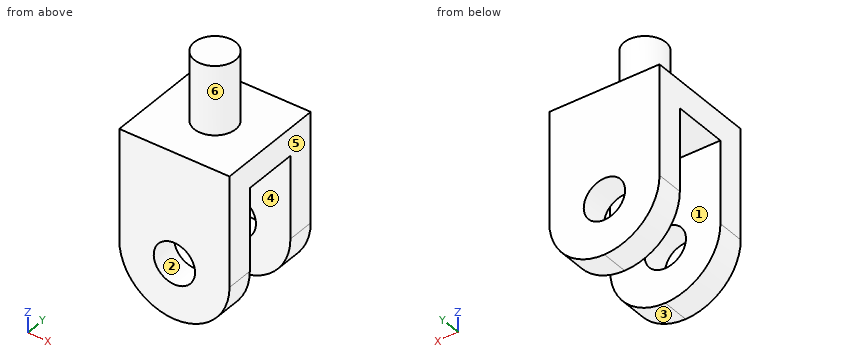
```python
from build123d import *

# Parameters (mm, degrees)
SKETCH1_W           = 16
SKETCH1_H           = 16
BOSS_EXTRUDE1_DEPTH = 24
SKETCH3_R           = 3
BOSS_EXTRUDE2_DEPTH = 10
SKETCH4_W           = 20
SKETCH4_H           = 8
CUT_EXTRUDE1_DEPTH  = 39.418745425
SKETCH5_R           = 3
CUT_EXTRUDE2_DEPTH  = 39.418745425
FILLET1_R           = 8


with BuildPart() as part:
    # Sketch1 → Boss-Extrude1 (new body)
    with BuildSketch(Plane.XY):
        Rectangle(SKETCH1_W, SKETCH1_H)
    extrude(amount=BOSS_EXTRUDE1_DEPTH)

    # Sketch3 → Boss-Extrude2 (add)
    with BuildSketch(Plane.XY.offset(24)):
        Circle(SKETCH3_R)
    extrude(amount=BOSS_EXTRUDE2_DEPTH)

    # Sketch4 → Cut-Extrude1 (cut, through all)
    with BuildSketch(Plane.ZY.offset(8)):
        with Locations((10, 0)):
            Rectangle(SKETCH4_W, SKETCH4_H)
    extrude(amount=-CUT_EXTRUDE1_DEPTH, mode=Mode.SUBTRACT)

    # Sketch5 → Cut-Extrude2 (cut, through all)
    with BuildSketch(Plane.XZ.offset(8)):
        with Locations(Location((0, 8, 0), (0, 0, 270))):
            Circle(SKETCH5_R)
    extrude(amount=-CUT_EXTRUDE2_DEPTH, mode=Mode.SUBTRACT)

    # Fillet1
    fillet1_edges = [part.edges().sort_by_distance(p)[0] for p in [
        (-8, 6, 0),
        (8, 6, 0),
        (8, -6, 0),
        (-8, -6, 0),
    ]]
    fillet(fillet1_edges, radius=FILLET1_R - 0.0001)  # a hair under: the kernel refuses the full size


solid = part.part
```
The model under review builds one solid part; all positions refer to its coordinate system, in mm. Face numbers are marked on the shaded views. A direction names the side the tool comes from. Round coordinates to 2 decimals unless told otherwise and drop trailing zeros. Write each loop counter-clockwise with the first axis right and the second up, starting at its lowest first coordinate (ties: lowest second). Pieces come first, ordered by that corner, then holes.
(1) Wall thickness on L1, parallel to X at y = 5.85, z = 8; L2, parallel to Y at x = 6, z = 6; L3, parallel to Z at x = -5, y = -2.75: over which ranges is each line inside the solid? List them lowest first.
(2) Machinability: for the marked faces 4, 5 and 6, which of the approach directions +Z, -Z, +X, -X, +Y, -Y give a long, thin tool a straight path to every point of the face, cutting with its end or side? Answer none if there is none.
(3) We need section C-C on z = 7.5. Give the boundary of the cut face in (x, y), and give its area (3 significant figures).
(4) Mouldability with a two-part tool opening along Z and no side actions: class the marked faces 1, 2 and 3 as +Z half, -Z half, draft (parallel to the pull), parting line (faces both ways), or undercut.
(5) Insertion check: pin 1 (7 mm diameter, centred on x = 0, z = 8, fed in from +Y); pin 2 (4 mm diameter, centred on x = -1.5, y = 1, fed in from -Z). Each pin has a flat end and moves straight along its axis. Give the tip position at first contact, or say it passes through.
(6) We need section D-D on x = -2.5. Give the boundary of the cut face in (y, z), and give its area (3 significant figures).
(7) We need section A-A on z = 2. Give the boundary of the cut face in (x, y), and give its area (3 significant figures).
Findings below:
1. L1: x = -8 to -3, 3 to 8
1. L2: y = -8 to -4, 4 to 8
1. L3: z = 20 to 24
2. face 4: -Z, +X, -X
2. face 5: +Z, -Z, +X, +Y, -Y
2. face 6: +Z
3. outline: (-7.98, -8) - (-2.96, -8) - (-2.96, -4) - (-7.98, -4) - close; (-7.98, 4) - (-2.96, 4) - (-2.96, 8) - (-7.98, 8) - close; (2.96, -8) - (7.98, -8) - (7.98, -4) - (2.96, -4) - close; (2.96, 4) - (7.98, 4) - (7.98, 8) - (2.96, 8) - close
3. area: 80.4 mm2
4. face 1: draft
4. face 2: undercut
4. face 3: -Z half
5. pin 1: stops at y = 8
5. pin 2: stops at z = 20
6. outline: (-8, 0.4) - (-4, 0.4) - (-4, 6.34) - (-8, 6.34) - close; (-8, 9.66) - (-4, 9.66) - (-4, 20) - (4, 20) - (4, 9.66) - (8, 9.66) - (8, 24) - (1.66, 24) - (1.66, 34) - (-1.66, 34) - (-1.66, 24) - (-8, 24) - close; (4, 0.4) - (8, 0.4) - (8, 6.34) - (4, 6.34) - close
6. area: 227 mm2
7. outline: (-5.29, -8) - (5.29, -8) - (5.29, -4) - (-5.29, -4) - close; (-5.29, 4) - (5.29, 4) - (5.29, 8) - (-5.29, 8) - close
7. area: 84.7 mm2
